Design review of the part built by this model. Coordinates are the model's own, in mm. Face numbers are marked on the shaded views. Coordinates: 2 decimals unless noted, no trailing zeros. Write each loop counter-clockwise with the first axis right and the second up, starting at its lowest first coordinate (ties: lowest second). Pieces come first, ordered by that corner, then holes. Notation, with made-up numbers: (-6, 87.5) -> (51, 87.5) arc R18 cw to (51, 103.5) -> close; hole circle Ø11 at (57.5, 41). An arc over 180 degrees is marked (long way). One line per question, with ' | ' between items. Start each with the question number.
Q1. Wall thickness on probe 1 along Y at (x, z) = (0, 0.6); probe 2 along Y at (x, z) = (0, 3); probe 3 along X at (y, z) = (-2.25, 3.2): over which ranges is each line inside the solid? List them lowest first.
Q2. Draft analysis for pull direction X (two halves, no side actions). For the marked faces 1, 2, 3 and 4, state which applies: pulls with the +X half, pulls with the -X half, needs draft (parallel to the pull), parting line crosses it, or undercut.
Q3. Add section D-D on y = 0. State the section outline as (x, z) points.
Q4. Add section B-B on x = 0. State the section outline as (y, z) points.
Q5. Add section C-C on z = 2.35. State the section outline as (x, y) points.
Q6. For P1, Ø2, axis at y = -6.5, z = 3.5, coming from the -X side; P2, Ø3, axis at x = 0, y = 0, coming from the +Z side, all flat-tipped, find the tip position at first contact; note any pin that passes through.
Q7. Add section A-A on y = 9. State the section outline as (x, z) points, and give its area (3 significant figures).
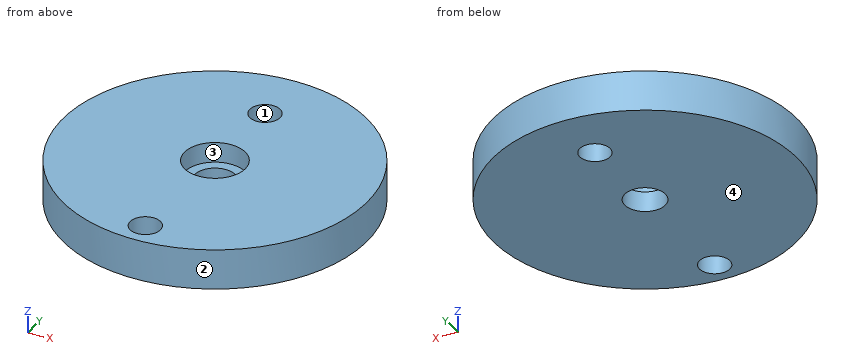
from build123d import *

# Parameters (mm, degrees)
SKETCH1_R           = 15
SKETCH1_R_2         = 3
SKETCH1_R_3         = 1.5
BOSS_EXTRUDE1_DEPTH = 4
SKETCH1_3_R         = 3
SKETCH1_3_R_2       = 2
BOSS_EXTRUDE2_DEPTH = 2


with BuildPart() as part:
    # Sketch1 → Boss-Extrude1 (new body)
    with BuildSketch(Plane.XY):
        Circle(SKETCH1_R)
        Circle(SKETCH1_R_2, mode=Mode.SUBTRACT)
        with Locations((0, -12.5)):
            Circle(SKETCH1_R_3, mode=Mode.SUBTRACT)
        with Locations((0, 9)):
            Circle(SKETCH1_R_3, mode=Mode.SUBTRACT)
    extrude(amount=BOSS_EXTRUDE1_DEPTH)

    # Sketch1_3 → Boss-Extrude2 (add)
    with BuildSketch(Plane.XY):
        Circle(SKETCH1_3_R)
        Circle(SKETCH1_3_R_2, mode=Mode.SUBTRACT)
    extrude(amount=BOSS_EXTRUDE2_DEPTH)


solid = part.part
Output values:
1) probe 1: y = -15 to -14, -11 to -2, 2 to 7.5, 10.5 to 15 | probe 2: y = -15 to -14, -11 to -3, 3 to 7.5, 10.5 to 15 | probe 3: x = -14.83 to -1.98, 1.98 to 14.83
2) face 1: undercut | face 2: parting line crosses it | face 3: undercut | face 4: needs draft
3) outline: (-15, 0) -> (-2, 0) -> (-2, 2) -> (-3, 2) -> (-3, 4) -> (-15, 4) -> close; (2, 0) -> (15, 0) -> (15, 4) -> (3, 4) -> (3, 2) -> (2, 2) -> close
4) outline: (-15, 0) -> (-14, 0) -> (-14, 4) -> (-15, 4) -> close; (-11, 0) -> (-2, 0) -> (-2, 2) -> (-3, 2) -> (-3, 4) -> (-11, 4) -> close; (2, 0) -> (7.5, 0) -> (7.5, 4) -> (3, 4) -> (3, 2) -> (2, 2) -> close; (10.5, 0) -> (15, 0) -> (15, 4) -> (10.5, 4) -> close
5) outline: circle Ø30 at (0, 0); hole circle Ø6 at (0, 0); hole circle Ø3 at (0, -12.5); hole circle Ø3 at (0, 9)
6) P1: stops at x = -13.96 | P2: passes through
7) outline: (-12, 0) -> (-1.5, 0) -> (-1.5, 4) -> (-12, 4) -> close; (1.5, 0) -> (12, 0) -> (12, 4) -> (1.5, 4) -> close | area: 84.0 mm2
